```python
from build123d import *

# Parameters (mm, degrees)
SKETCH1_R           = 3
BOSS_EXTRUDE2_DEPTH = 5


with BuildPart() as part:
    # Sketch1 → Boss-Extrude2 (new body)
    with BuildSketch(Plane(origin=(0, 0, 0), x_dir=(1, 0, 0), z_dir=(0, 1, 0))):
        with BuildLine():
            Line((-4.156921938, -0.6), (-20, -0.6))
            Line((-20, -0.6), (-20, 0.6))
            Line((-20, 0.6), (-4.156921938, 0.6))
            ThreePointArc((-4.156921938, 0.6), (-2.1, 3.637306696), (1.558845727, 3.9))
            Line((1.558845727, 3.9), (9.480384758, 17.620508076))
            Line((9.480384758, 17.620508076), (10.519615242, 17.020508076))
            Line((10.519615242, 17.020508076), (2.598076211, 3.3))
            ThreePointArc((2.598076211, 3.3), (4.2, 0), (2.598076211, -3.3))
            Line((2.598076211, -3.3), (10.519615242, -17.020508076))
            Line((10.519615242, -17.020508076), (9.480384758, -17.620508076))
            Line((9.480384758, -17.620508076), (1.558845727, -3.9))
            ThreePointArc((1.558845727, -3.9), (-2.1, -3.637306696), (-4.156921938, -0.6))
        make_face()
        with Locations(Location((0, 0, 0), (0, 0, 270))):
            Circle(SKETCH1_R, mode=Mode.SUBTRACT)
    extrude(amount=BOSS_EXTRUDE2_DEPTH)


solid = part.part
```
The listing builds one solid part. Answer for the finished solid, in the listing's coordinates (mm). A direction names the side the tool comes from. Round coordinates to 2 decimals unless told otherwise and drop trailing zeros. Loops run counter-clockwise (first coordinate to the right, second up) from the corner with the lowest first, then second, coordinate; pieces in that order, holes last.
1) For a pull along Z with two mould halves and no side action, classify faces 4 (the face through (-12, 2, -0.6)), 5 (the face through (0.9, 2.46, 2.86)), 6 (the face through (6.614, 2.465, -10.256)), 7 (the face through (10.007, 2.465, 17.316)) as released by +Z, released by -Z, zero draft, split by the parting line, or undercut.
Outcome:
face 4: released by -Z
face 5: undercut
face 6: undercut
face 7: released by +Z
2) A cutting plane is placed at A-A on x = 0. Determine the outline of the cut face in (y, z), plus the area to 3 significant figures.
Outcome:
outline: (0, -4.2) - (5, -4.2) - (5, -3) - (0, -3) - close; (0, 3) - (5, 3) - (5, 4.2) - (0, 4.2) - close
area: 12.0 mm2
3) A cutting plane is placed at B-B on z = 0. Determine the outline of the cut face in (x, y), plus the area to 3 significant figures.
Outcome:
outline: (-20, 0) - (-3, 0) - (-3, 5) - (-20, 5) - close; (3, 0) - (4.2, 0) - (4.2, 5) - (3, 5) - close
area: 91.0 mm2
4) A cutting plane is placed at D-D on x = -13.5. Determine the outline of the cut face in (y, z), plus the area to 3 significant figures.
Outcome:
outline: (0, -0.6) - (5, -0.6) - (5, 0.6) - (0, 0.6) - close
area: 6.00 mm2
5) A cutting plane is placed at C-C on y = 2.75. Determine the outline of the cut face in (x, z).
Outcome:
outline: (-20, -0.6) - (-4.16, -0.6) arc R4.2 ccw to (1.56, -3.9) - (9.48, -17.62) - (10.52, -17.02) - (2.6, -3.3) arc R4.2 ccw to (2.6, 3.3) - (10.52, 17.02) - (9.48, 17.62) - (1.56, 3.9) arc R4.2 ccw to (-4.16, 0.6) - (-20, 0.6) - close; hole circle Ø6 at (0, 0)
6) For faces 1 (the face through (6.5, 2.46, 10.06)), 2 (the face through (-12, 2, 0.6)), 3 (the face through (3.2, 5, -0.1)), determine the directions among +Z, -Z, +X, -X, +Y, -Y from which every point of the face is accessible in a straight line to the end or side of a thin tool.
Outcome:
face 1: +X, +Y, -Y
face 2: +Z, -X, +Y, -Y
face 3: +Z, -Z, +X, -X, +Y
7) Given P1, Ø2, axis at y = 4, z = 13, coming from the +X side; P2, Ø12, axis at x = 0.5, z = -11, coming from the -Y side; P3, Ø2, axis at y = 0.5, z = -2.5, coming from the -X side; P4, Ø2, axis at y = 2.5, z = 6, coming from the -X side, each flat-ended and moving along its own axis, determine where each tip first touches the part or whether it passes through.
Outcome:
P1: stops at x = 8.78
P2: stops at y = 0
P3: stops at x = -3.92
P4: stops at x = 2.19
8) Consider line 1 (X direction, y = 3.1, z = 0); line 2 (Z direction, x = 9, y = 1.5); line 3 (Z direction, x = 1, y = 4). Determine where each line is inside the solid, lowest interval first.
Outcome:
line 1: x = -20 to -3, 3 to 4.2
line 2: z = -16.79 to -14.39, 14.39 to 16.79
line 3: z = -4.08 to -2.83, 2.83 to 4.08
